CAD build for the part. Positions are in the model's coordinates, mm. Face numbers are marked on the shaded views. A direction names the side the tool comes from. Give positions to 0.01 mm unless a question says otherwise; leave off trailing zeros. Loops run counter-clockwise (first coordinate to the right, second up) from the corner with the lowest first, then second, coordinate; pieces in that order, holes last. Notation, with made-up numbers: (79, 34) - (104, 34) arc R9 ccw to (104, 48) - close; hole circle Ø3 at (71.5, 62). An arc over 180 degrees is marked (long way). Return JSON: item names as keys, results as strings.
from build123d import *

# Parameters (mm, degrees)
SKETCH1_R           = 14.949572774
SKETCH1_R_2         = 2.099903903
BOSS_EXTRUDE1_DEPTH = 7.5
SKETCH2_R           = 14.949572774
BOSS_EXTRUDE2_DEPTH = 5
BOSS_EXTRUDE3_DEPTH = 1
BOSS_EXTRUDE4_DEPTH = 25
SKETCH5_R           = 2.099903903
CUT_EXTRUDE1_DEPTH  = 7
CHAMFER2_SIZE       = 0.5
CHAMFER3_SIZE       = 0.5


with BuildPart() as part:
    # Sketch1 → Boss-Extrude1 (new body)
    with BuildSketch(Plane.XY):
        Circle(SKETCH1_R)
        with Locations((9.999999776, -1e-09)):
            Circle(SKETCH1_R_2, mode=Mode.SUBTRACT)
        with Locations((-9.999999776, 1e-09)):
            Circle(SKETCH1_R_2, mode=Mode.SUBTRACT)
    extrude(amount=-BOSS_EXTRUDE1_DEPTH)

    # Sketch2 → Boss-Extrude2 (add)
    with BuildSketch(Plane(origin=(0, 0, -7.5), x_dir=(-1, 0, 0), z_dir=(0, 0, -1))):
        Circle(SKETCH2_R)
    extrude(amount=BOSS_EXTRUDE2_DEPTH)

    # Sketch3 → Boss-Extrude3 (add)
    with BuildSketch(Plane(origin=(0, 0, -12.5), x_dir=(-1, 0, 0), z_dir=(0, 0, -1))):
        with BuildLine():
            Line((-1e-09, 14.949572774), (-1e-09, -14.949572774))
            ThreePointArc((-1e-09, -14.949572774), (14.949572774, 0), (-1e-09, 14.949572774))
        make_face()
    extrude(amount=BOSS_EXTRUDE3_DEPTH)

    # Sketch4 → Boss-Extrude4 (add)
    with BuildSketch(Plane(origin=(0, 0, -12.5), x_dir=(-1, 0, 0), z_dir=(0, 0, -1))):
        with BuildLine():
            Line((-6.499816063, 13.462619257), (-6.499816063, -13.462619257))
            ThreePointArc((-6.499816063, -13.462619257), (-14.949572774, 0), (-6.499816063, 13.462619257))
        make_face()
    extrude(amount=BOSS_EXTRUDE4_DEPTH)

    # Sketch5 → Cut-Extrude1 (cut)
    with BuildSketch(Plane(origin=(0, 0, -37.5), x_dir=(-1, 0, 0), z_dir=(0, 0, -1))):
        with Locations((-9.999999776, -1e-09)):
            Circle(SKETCH5_R)
    extrude(amount=-CUT_EXTRUDE1_DEPTH, mode=Mode.SUBTRACT)

    # Chamfer2
    chamfer2_edges = [part.edges().sort_by_distance(p)[0] for p in [
        (14.949572774, 0, -37.5),
    ]]
    chamfer(chamfer2_edges, length=CHAMFER2_SIZE)

    # Chamfer3
    chamfer3_edges = [part.edges().sort_by_distance(p)[0] for p in [
        (-14.949572774, 0, 0),
    ]]
    chamfer(chamfer3_edges, length=CHAMFER3_SIZE)


solid = part.part
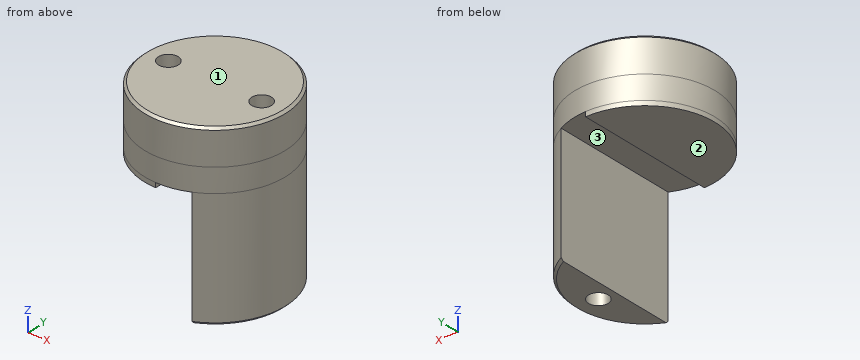
1. Cut at B-B, the plane z = -9. Write the cut outline in (x, y).
Values follow:
{"outline": "circle Ø29.9 at (0, 0)"}
2. Drill centre lines: probe 1 along X at (y, z) = (0, -33.75); probe 2 along X at (y, z) = (-0.75, -3.5); probe 3 along Y at (x, z) = (10, -2.5). Where is each one in solid material? Low to high.
Values follow:
{"probe 1": "x = 6.5 to 7.9, 12.1 to 14.95", "probe 2": "x = -14.93 to -11.96, -8.04 to 8.04, 11.96 to 14.93", "probe 3": "y = -11.11 to -2.1, 2.1 to 11.11"}
3. Cut at A-A, the plane z = -14. Write the cut outline in (x, y), plus the area to 3 significant figures.
Values follow:
{"outline": "(6.5, -13.46) arc R14.95 ccw to (6.5, 13.46) - close", "area": "163 mm²"}
4. Which spindle directions (+Z, -Z, +X, -X, +Y, -Y) get a long thin tool onto all of the face, cutting with end or side? Do the marked faces 1, 2 and 3. Say none if no direction does.
Values follow:
{"face 1": "+Z, +X, -X, +Y, -Y", "face 2": "-Z, -X, +Y, -Y", "face 3": "-Z, +Y, -Y"}
5. Drop flat-ended pins along their axis: P1, Ø12, axis at x = -5.5, y = 3.5, coming from the -Z side; P2, Ø10, axis at y = -5.5, z = -18.5, coming from the +X side; P3, Ø6.5, axis at x = 10, y = 0, coming from the -Z side; P4, Ø7.5, axis at y = 1.5, z = -25, coming from the -X side. Give the stop position or say it passes through.
Values follow:
{"P1": "stops at z = -13.5", "P2": "stops at x = 14.94", "P3": "stops at z = -37.5", "P4": "stops at x = 6.5"}
